Source: CAD feature listing. Evaluate the final solid. Frame: model axes, mm. Face numbers are marked on the shaded views. A direction names the side the tool comes from. Coordinates: 2 decimals unless noted, no trailing zeros. Order: outer loops, then holes, each group sorted by start corner. A loop starts at its lowest first (then second) coordinate and runs counter-clockwise, first axis right, second up. Notation, with made-up numbers: (88, -34) - (104, -34) arc R23 ccw to (104, -12) - close; hole circle Ø7 at (42, 77). An arc over 180 degrees is marked (long way). One line per question, with ' | ' between items. Start each with the question number.
(1) Line query: line 1 along X through (y, z) = (-41, -0.4); line 2 along X through (y, z) = (-41, 14.25); line 3 along X through (y, z) = (-12, 10). Output: solid intervals per line, ascending.
(2) Section B-B (y = -5). Return the cut outline in (x, z).
(3) Access query for the marked faces 4 and 5. Directions: +Z, -Z, +X, -X, +Y, -Y. A direction counts if a zero-diameter tool reaches every point of the face in a straight line with its end or side. Return the directions, or none.
(4) Contact query for flat-ended pins moving along their axis: P1, Ø4, axis at x = -6, y = -25, coming from the +Z side; P2, Ø8, axis at y = -31, z = 2.5, coming from the +X side; P3, Ø0.8, axis at y = -45.5, z = 9.5, coming from the -X side; P4, Ø3, axis at x = -19.46, y = -41, coming from the -Z side. Output: stop coordinate, or through.
(5) Draft query along X for the marked faces 1, 2 and 3. Return one class per face: +X half, -X half, draft (parallel to the pull), parting line (faces both ways), or undercut.
(6) Section A-A (z = 6.25). Return the cut outline in (x, y).
(7) Section D-D (x = 10.5). Return the cut outline in (y, z).
(8) Section C-C (y = -35). Return the cut outline in (x, z).
from build123d import *

# Parameters (mm, degrees)
F1_DEPTH      = 46
F3_R          = 1.6
F4_DEPTH      = 24
F5_DEPTH      = 24.001
F5_DEPTH_BACK = 3.001
F6_DEPTH      = 25
F7_DEPTH      = 2
F8_DEPTH      = 25
F9_DEPTH      = 1


with BuildPart() as f1:
    # F0 (on Front) → F1 (new body)
    with BuildSketch(Plane.XZ):
        with BuildLine():
            Line((16.5, 0), (-16.5, 0))
            Line((-16.5, 0), (-16.5, 21))
            Line((-16.5, 21), (-16.5, 24))
            Line((-16.5, 24), (-19.5, 24))
            Line((-19.5, 24), (-19.5, 2))
            ThreePointArc((-19.5, 2), (-18.035534, -1.535534), (-14.5, -3))
            Line((-14.5, -3), (14.5, -3))
            ThreePointArc((14.5, -3), (18.035534, -1.535534), (19.5, 2))
            Line((19.5, 2), (19.5, 24))
            Line((19.5, 24), (16.5, 24))
            Line((16.5, 24), (16.5, 21))
            Line((16.5, 21), (16.5, 0))
        make_face()
    extrude(amount=F1_DEPTH)

    # F3 (on Top) → F4 (join, through all)
    with BuildSketch(Plane.XY):
        with BuildLine():
            ThreePointArc((-16.511744, -2.294334), (-23.457821, -5), (-16.511744, -7.705666))
            Line((-16.511744, -7.705666), (-16.511744, -2.294334))
        make_face()
        with Locations((-19.457821, -5)):
            Circle(F3_R, mode=Mode.SUBTRACT)
        with BuildLine():
            Line((16.511744, -2.294334), (16.511744, -7.705666))
            ThreePointArc((16.511744, -7.705666), (23.457821, -5), (16.511744, -2.294334))
        make_face()
        with Locations((19.457821, -5)):
            Circle(F3_R, mode=Mode.SUBTRACT)
        with BuildLine():
            Line((16.511744, -38.294334), (16.511744, -43.705666))
            ThreePointArc((16.511744, -43.705666), (23.457821, -41), (16.511744, -38.294334))
        make_face()
        with Locations((19.457821, -41)):
            Circle(F3_R, mode=Mode.SUBTRACT)
        with BuildLine():
            ThreePointArc((-16.511744, -38.294334), (-23.457821, -41), (-16.511744, -43.705666))
            Line((-16.511744, -43.705666), (-16.511744, -38.294334))
        make_face()
        with Locations((-19.457821, -41)):
            Circle(F3_R, mode=Mode.SUBTRACT)
    extrude(amount=F4_DEPTH)

    # F3 (on Top) → F5 (cut, two sides)
    with BuildSketch(Plane.XY) as f5_sk:
        with Locations((19.457821, -5)):
            Circle(F3_R)
        with Locations((-19.457821, -5)):
            Circle(F3_R)
        with Locations((-19.457821, -41)):
            Circle(F3_R)
        with Locations((19.457821, -41)):
            Circle(F3_R)
    extrude(amount=F5_DEPTH, mode=Mode.SUBTRACT)
    extrude(f5_sk.sketch, amount=-F5_DEPTH_BACK, mode=Mode.SUBTRACT)

    # F3 (on Top) → F6 (cut)
    with BuildSketch(Plane.XY):
        with BuildLine():
            Line((16.511744, -2.294334), (16.511744, -7.705666))
            ThreePointArc((16.511744, -7.705666), (23.457821, -5), (16.511744, -2.294334))
        make_face()
        with Locations((19.457821, -5)):
            Circle(F3_R, mode=Mode.SUBTRACT)
        with BuildLine():
            ThreePointArc((-16.511744, -2.294334), (-23.457821, -5), (-16.511744, -7.705666))
            Line((-16.511744, -7.705666), (-16.511744, -2.294334))
        make_face()
        with Locations((-19.457821, -5)):
            Circle(F3_R, mode=Mode.SUBTRACT)
        with BuildLine():
            Line((16.511744, -38.294334), (16.511744, -43.705666))
            ThreePointArc((16.511744, -43.705666), (23.457821, -41), (16.511744, -38.294334))
        make_face()
        with Locations((19.457821, -41)):
            Circle(F3_R, mode=Mode.SUBTRACT)
    extrude(amount=-F6_DEPTH, mode=Mode.SUBTRACT)

    # F3 (on Top) → F7 (join)
    with BuildSketch(Plane.XY):
        with BuildLine():
            ThreePointArc((-16.511744, -38.294334), (-23.457821, -41), (-16.511744, -43.705666))
            Line((-16.511744, -43.705666), (-16.511744, -38.294334))
        make_face()
        with Locations((-19.457821, -41)):
            Circle(F3_R, mode=Mode.SUBTRACT)
        with BuildLine():
            ThreePointArc((-16.511744, -2.294334), (-23.457821, -5), (-16.511744, -7.705666))
            Line((-16.511744, -7.705666), (-16.511744, -2.294334))
        make_face()
        with Locations((-19.457821, -5)):
            Circle(F3_R, mode=Mode.SUBTRACT)
        with BuildLine():
            Line((16.511744, -38.294334), (16.511744, -43.705666))
            ThreePointArc((16.511744, -43.705666), (23.457821, -41), (16.511744, -38.294334))
        make_face()
        with Locations((19.457821, -41)):
            Circle(F3_R, mode=Mode.SUBTRACT)
        with BuildLine():
            Line((16.511744, -2.294334), (16.511744, -7.705666))
            ThreePointArc((16.511744, -7.705666), (23.457821, -5), (16.511744, -2.294334))
        make_face()
        with Locations((19.457821, -5)):
            Circle(F3_R, mode=Mode.SUBTRACT)
    extrude(amount=-F7_DEPTH)

    # F3 (on Top) → F8 (cut)
    with BuildSketch(Plane.XY):
        with BuildLine():
            Line((16.511744, -2.294334), (16.511744, -7.705666))
            ThreePointArc((16.511744, -7.705666), (23.457821, -5), (16.511744, -2.294334))
        make_face()
        with Locations((19.457821, -5)):
            Circle(F3_R, mode=Mode.SUBTRACT)
        with BuildLine():
            ThreePointArc((16.511744, -2.294334), (15.457821, -5), (16.511744, -7.705666))
            Line((16.511744, -7.705666), (16.511744, -2.294334))
        make_face()
        with BuildLine():
            Line((16.511744, -38.294334), (16.511744, -43.705666))
            ThreePointArc((16.511744, -43.705666), (23.457821, -41), (16.511744, -38.294334))
        make_face()
        with Locations((19.457821, -41)):
            Circle(F3_R, mode=Mode.SUBTRACT)
        with BuildLine():
            ThreePointArc((16.511744, -38.294334), (15.457821, -41), (16.511744, -43.705666))
            Line((16.511744, -43.705666), (16.511744, -38.294334))
        make_face()
        with BuildLine():
            ThreePointArc((-16.511744, -2.294334), (-23.457821, -5), (-16.511744, -7.705666))
            Line((-16.511744, -7.705666), (-16.511744, -2.294334))
        make_face()
        with Locations((-19.457821, -5)):
            Circle(F3_R, mode=Mode.SUBTRACT)
        with BuildLine():
            Line((-16.511744, -2.294334), (-16.511744, -7.705666))
            ThreePointArc((-16.511744, -7.705666), (-15.457821, -5), (-16.511744, -2.294334))
        make_face()
        with BuildLine():
            ThreePointArc((-16.511744, -38.294334), (-23.457821, -41), (-16.511744, -43.705666))
            Line((-16.511744, -43.705666), (-16.511744, -38.294334))
        make_face()
        with Locations((-19.457821, -41)):
            Circle(F3_R, mode=Mode.SUBTRACT)
        with BuildLine():
            Line((-16.511744, -38.294334), (-16.511744, -43.705666))
            ThreePointArc((-16.511744, -43.705666), (-15.457821, -41), (-16.511744, -38.294334))
        make_face()
    extrude(amount=-F8_DEPTH, mode=Mode.SUBTRACT)

    # F3 (on Top) → F9 (join)
    with BuildSketch(Plane.XY):
        with BuildLine():
            Line((-16.511744, -38.294334), (-16.511744, -43.705666))
            ThreePointArc((-16.511744, -43.705666), (-15.457821, -41), (-16.511744, -38.294334))
        make_face()
        with BuildLine():
            ThreePointArc((-16.511744, -38.294334), (-23.457821, -41), (-16.511744, -43.705666))
            Line((-16.511744, -43.705666), (-16.511744, -38.294334))
        make_face()
        with Locations((-19.457821, -41)):
            Circle(F3_R, mode=Mode.SUBTRACT)
        with BuildLine():
            ThreePointArc((16.511744, -38.294334), (15.457821, -41), (16.511744, -43.705666))
            Line((16.511744, -43.705666), (16.511744, -38.294334))
        make_face()
        with BuildLine():
            Line((16.511744, -38.294334), (16.511744, -43.705666))
            ThreePointArc((16.511744, -43.705666), (23.457821, -41), (16.511744, -38.294334))
        make_face()
        with Locations((19.457821, -41)):
            Circle(F3_R, mode=Mode.SUBTRACT)
        with BuildLine():
            ThreePointArc((16.511744, -2.294334), (15.457821, -5), (16.511744, -7.705666))
            Line((16.511744, -7.705666), (16.511744, -2.294334))
        make_face()
        with BuildLine():
            Line((16.511744, -2.294334), (16.511744, -7.705666))
            ThreePointArc((16.511744, -7.705666), (23.457821, -5), (16.511744, -2.294334))
        make_face()
        with Locations((19.457821, -5)):
            Circle(F3_R, mode=Mode.SUBTRACT)
        with BuildLine():
            Line((-16.511744, -2.294334), (-16.511744, -7.705666))
            ThreePointArc((-16.511744, -7.705666), (-15.457821, -5), (-16.511744, -2.294334))
        make_face()
        with BuildLine():
            ThreePointArc((-16.511744, -2.294334), (-23.457821, -5), (-16.511744, -7.705666))
            Line((-16.511744, -7.705666), (-16.511744, -2.294334))
        make_face()
        with Locations((-19.457821, -5)):
            Circle(F3_R, mode=Mode.SUBTRACT)
    extrude(amount=-F9_DEPTH)


solid = f1.part
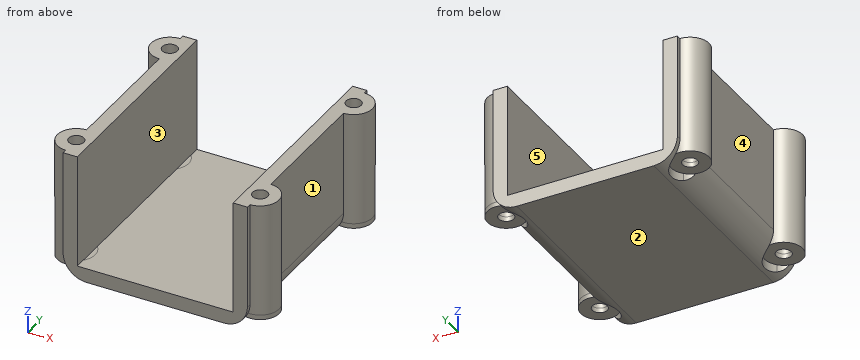
Response values:
1) line 1: x = -23.46 to -21.06, -17.86 to 17.86, 21.06 to 23.46 | line 2: x = -23.46 to -21.06, -17.86 to -16.5, 16.5 to 17.86, 21.06 to 23.46 | line 3: x = -19.5 to -16.5, 16.5 to 19.5
2) outline: (-23.46, -1) - (-21.06, -1) - (-21.06, 24) - (-23.46, 24) - close; (-17.86, -1) - (-15.46, -1) - (-15.46, -2.91) arc R5 ccw to (-14.5, -3) - (14.5, -3) arc R5 ccw to (15.46, -2.91) - (15.46, -1) - (17.86, -1) - (17.86, 24) - (16.5, 24) - (16.5, 0) - (-16.5, 0) - (-16.5, 24) - (-17.86, 24) - close; (21.06, -1) - (23.46, -1) - (23.46, 24) - (21.06, 24) - close
3) face 4: +Z, -Z, -X | face 5: +Z, +Y, -Y
4) P1: stops at z = 0 | P2: stops at x = 19.5 | P3: stops at x = -19.5 | P4: passes through
5) face 1: +X half | face 2: draft | face 3: undercut
6) outline: (-19.5, -46) - (-16.5, -46) - (-16.5, 0) - (-19.5, 0) - (-19.5, -1) arc R4 ccw to (-19.5, -9) - (-19.5, -37) arc R4 ccw to (-19.5, -45) - close; (16.5, -46) - (19.5, -46) - (19.5, -45) arc R4 ccw to (19.5, -37) - (19.5, -9) arc R4 ccw to (19.5, -1) - (19.5, 0) - (16.5, 0) - close; hole circle Ø3.2 at (-19.46, -41); hole circle Ø3.2 at (-19.46, -5); hole circle Ø3.2 at (19.46, -41); hole circle Ø3.2 at (19.46, -5)
7) outline: (-46, -3) - (0, -3) - (0, 0) - (-46, 0) - close
8) outline: (-19.5, 2) arc R5 ccw to (-14.5, -3) - (14.5, -3) arc R5 ccw to (19.5, 2) - (19.5, 24) - (16.5, 24) - (16.5, 0) - (-16.5, 0) - (-16.5, 24) - (-19.5, 24) - close
